```python
from build123d import *

# Parameters (mm, degrees)
SKETCH1_R           = 10
BOSS_EXTRUDE1_DEPTH = 300
SKETCH2_R           = 8.5
BOSS_EXTRUDE2_DEPTH = 5
SKETCH6_R           = 10
CUT_EXTRUDE2_DEPTH  = 24
SKETCH7_W           = 5
SKETCH7_H           = 5
CUT_EXTRUDE3_DEPTH  = 40
SKETCH10_R          = 12.5
BOSS_EXTRUDE4_DEPTH = 15


with BuildPart() as part:
    # Sketch1 → Boss-Extrude1 (new body)
    with BuildSketch(Plane(origin=(0, 0, 0), x_dir=(0, 0, -1), z_dir=(1, 0, 0))):
        Circle(SKETCH1_R)
    extrude(amount=BOSS_EXTRUDE1_DEPTH)

    # Sketch2 → Boss-Extrude2 (add)
    with BuildSketch(Plane(origin=(300, 0, 0), x_dir=(0, 0, -1), z_dir=(1, 0, 0))):
        Circle(SKETCH2_R)
    extrude(amount=BOSS_EXTRUDE2_DEPTH)

    # Sketch6 → Cut-Extrude2 (cut)
    with BuildSketch(Plane.ZY):
        Circle(SKETCH6_R)
        with BuildLine():
            Line((-2.5, 7.071067812), (-2.5, 5))
            Line((-2.5, 5), (2.5, 5))
            Line((2.5, 5), (2.5, 7.071067812))
            ThreePointArc((2.5, 7.071067812), (0, -7.5), (-2.5, 7.071067812))
        make_face(mode=Mode.SUBTRACT)
    extrude(amount=-CUT_EXTRUDE2_DEPTH, mode=Mode.SUBTRACT)

    # Sketch7 → Cut-Extrude3 (cut)
    with BuildSketch(Plane(origin=(305, 0, 0), x_dir=(0, 0, -1), z_dir=(1, 0, 0))):
        with Locations((0, 8.5)):
            Rectangle(SKETCH7_W, SKETCH7_H)
    extrude(amount=-CUT_EXTRUDE3_DEPTH, mode=Mode.SUBTRACT)

    # Sketch10 → Boss-Extrude4 (add)
    with BuildSketch(Plane(origin=(225, 0, 0), x_dir=(0, 0, -1), z_dir=(1, 0, 0))):
        Circle(SKETCH10_R)
    extrude(amount=-BOSS_EXTRUDE4_DEPTH)


solid = part.part
```
Input: part model. Units: mm. Frame: model coordinates. A direction names the side the tool comes from. Coordinates: 2 decimals unless noted, no trailing zeros. Loops run counter-clockwise (first coordinate to the right, second up) from the corner with the lowest first, then second, coordinate; pieces in that order, holes last. Notation, with made-up numbers: (12, 67.5) -> (39, 67.5) arc R23 ccw to (39, 77.5) -> close; hole circle Ø4 at (70, 44.25). An arc over 180 degrees is marked (long way). Use a Markdown table: item, result.
1) Material intervals for line 1 along X through (y, z) = (3, -9.75); line 2 along Y through (x, z) = (85.5, 0.25); line 3 along Z through (x, y) = (291.5, -1), sorted ascending. Write a range as from..to.
Results found:
| item | result |
|---|---|
| line 1 | x = 210..225 |
| line 2 | y = -10..10 |
| line 3 | z = -9.95..9.95 |
2) Pull-direction query (Z, two-part tool) for faces 1 (the flat face through (0, 0, 0)), 2 (the flat face through (12, 5, 0)), 3 (the cylindrical face through (217.605, 3.755, -11.923)); classes: released by +Z, released by -Z, zero draft, split by the parting line, or undercut.
Results found:
| item | result |
|---|---|
| face 1 | zero draft |
| face 2 | undercut |
| face 3 | split by the parting line |
3) Cut plane B-B (y = 0). Return the cut outline in (x, z), then the cut area to 3 significant figures.
Results found:
| item | result |
|---|---|
| outline | (0, -7.5) -> (24, -7.5) -> (24, -10) -> (210, -10) -> (210, -12.5) -> (225, -12.5) -> (225, -10) -> (300, -10) -> (300, -8.5) -> (305, -8.5) -> (305, 8.5) -> (300, 8.5) -> (300, 10) -> (225, 10) -> (225, 12.5) -> (210, 12.5) -> (210, 10) -> (24, 10) -> (24, 7.5) -> (0, 7.5) -> close |
| area | 6,040 mm2 |
4) Cut plane C-C (x = 184.5). Return the cut outline in (y, z), then the cut area to 3 significant figures.
Results found:
| item | result |
|---|---|
| outline | circle Ø20 at (0, 0) |
| area | 314 mm2 |
5) Access query for faces 4 (the flat face through (225, 10.2, 0.1)), 5 (the flat face through (305, 0, 0)), 6 (the flat face through (285, 6, 0)), 7 (the cylindrical face through (11.832, -7.494, 0.294)). Directions: +Z, -Z, +X, -X, +Y, -Y. A direction counts if a zero-diameter tool reaches every point of the face in a straight line with its end or side. Return the directions, or none.
Results found:
| item | result |
|---|---|
| face 4 | +X |
| face 5 | +Z, -Z, +X, +Y, -Y |
| face 6 | +X, +Y |
| face 7 | -X |
6) Cut plane A-A (z = 0). Return the cut outline in (x, y).
Results found:
| item | result |
|---|---|
| outline | (0, -7.5) -> (24, -7.5) -> (24, -10) -> (210, -10) -> (210, -12.5) -> (225, -12.5) -> (225, -10) -> (300, -10) -> (300, -8.5) -> (305, -8.5) -> (305, 6) -> (265, 6) -> (265, 10) -> (225, 10) -> (225, 12.5) -> (210, 12.5) -> (210, 10) -> (24, 10) -> (24, 5) -> (0, 5) -> close |
7) Contact query for flat-ended pins moving along their axis: pin 1 (4 mm diameter, centred on x = 294.5, y = 8, fed in from +Z); pin 2 (6 mm diameter, centred on x = 234, y = 9, fed in from -Z); pin 3 (4 mm diameter, centred on x = 282, y = 7.5, fed in from -Z); pin 4 (6 mm diameter, centred on y = -3.5, z = -1, fed in from -X). Output: stop coordinate, or through.
Results found:
| item | result |
|---|---|
| pin 1 | stops at z = 8 |
| pin 2 | stops at z = -8 |
| pin 3 | stops at z = -8.35 |
| pin 4 | stops at x = 0 |
